```python
from build123d import *

# Parameters (mm, degrees)
CYLINDER003_R     = 2.5
CYLINDER003_DEPTH = 10
CYLINDER_R        = 5
CYLINDER_DEPTH    = 10
CYLINDER002_R     = 2.5
CYLINDER002_DEPTH = 10


with BuildPart() as cylinder003:
    # Cylinder003 → Cylinder003 (new body)
    with BuildSketch(Plane(origin=(-5, 0, 0), x_dir=(0, 0, -1), z_dir=(1, 0, 0))):
        Circle(CYLINDER003_R)
    extrude(amount=CYLINDER003_DEPTH)


with BuildPart() as cut001:
    # Cylinder → Cylinder (new body)
    with BuildSketch(Plane(origin=(-5, 0, 0), x_dir=(0, 0, -1), z_dir=(1, 0, 0))):
        Circle(CYLINDER_R)
    extrude(amount=CYLINDER_DEPTH)

    # Cut001: cut Cylinder003
    add(cylinder003.part, mode=Mode.SUBTRACT)


with BuildPart() as cylinder002:
    # Cylinder002 → Cylinder002 (new body)
    with BuildSketch(Plane(origin=(-5, 0, 0), x_dir=(0, 0, -1), z_dir=(1, 0, 0))):
        Circle(CYLINDER002_R)
    extrude(amount=CYLINDER002_DEPTH)


with BuildPart() as fusion:
    # Sketch → Revolve (revolve)
    with BuildSketch(Plane.XY):
        Polygon((-4.4, 0), (-4.4, 7.615), (-3, 9.015), (3, 9.015), (4.4, 7.615), (4.4, 0), (0, 0), align=None)
    revolve(axis=Axis((0, 0, 0), (1, 0, 0)))

    # Cut: cut Cylinder002
    add(cylinder002.part, mode=Mode.SUBTRACT)

    # Fusion: union Cut001
    add(cut001.part)


solid = fusion.part
```
Geometry: final body of the model. Coordinates: model frame, mm. A direction names the side the tool comes from. Coordinates: 2 decimals unless noted, no trailing zeros. Order: outer loops, then holes, each group sorted by start corner. A loop starts at its lowest first (then second) coordinate and runs counter-clockwise, first axis right, second up. Notation, with made-up numbers: (32.5, 26) - (73.5, 26) arc R18 ccw to (73.5, 61) - close; hole circle Ø11 at (10.25, 21). An arc over 180 degrees is marked (long way). Write each question's results on one line, items separated by ' | '.
1) Section D-D, the plane x = 3.75. Return loops of the section in (y, z) (3 decimals).
Results list:
outline: circle Ø16.53 at (0, 0); hole circle Ø5 at (0, 0)
2) Pull-direction query (Y, two-part tool) for faces 1 (the cylindrical face through (0.04, -7.15, -5.49)), 2 (the cylindrical face through (-0.07, -2.44, 0.54)), 3 (the flat face through (4.4, 2, -5)); classes: pulls with the +Y half, pulls with the -Y half, needs draft (parallel to the pull), parting line crosses it, or undercut.
Results list:
face 1: parting line crosses it | face 2: undercut | face 3: needs draft
3) Section A-A, the plane y = 0. Return loops of the section in (x, z) (3 decimals), plus the area to 3 significant figures.
Results list:
outline: (-5, -5) - (-4.4, -5) - (-4.4, -7.615) - (-3, -9.015) - (3, -9.015) - (4.4, -7.615) - (4.4, -5) - (5, -5) - (5, -2.5) - (-5, -2.5) - close; (-5, 2.5) - (5, 2.5) - (5, 5) - (4.4, 5) - (4.4, 7.615) - (3, 9.015) - (-3, 9.015) - (-4.4, 7.615) - (-4.4, 5) - (-5, 5) - close | area: 117 mm^2
4) Set-up query: faces 4 (the flat face through (-5, -2, -2)), 5 (the cylindrical face through (4.7, -4.88, 1.08)), 6 (the flat face through (-4.4, -2, -5)). Return all of +Z, -Z, +X, -X, +Y, -Y with unobstructed straight access to the full face (end or side cutting, diameter ignored); none if empty.
Results list:
face 4: +Z, -Z, -X, +Y, -Y | face 5: +X | face 6: -X
5) Section C-C, the plane x = 2. Return loops of the section in (y, z) (3 decimals).
Results list:
outline: circle Ø18.03 at (0, 0); hole circle Ø5 at (0, 0)
6) Line query: line 1 (Y direction, x = -4.5, z = 4); line 2 (X direction, y = 5.5, z = 1.25); line 3 (Y direction, x = -3.5, z = 0.75). Output: solid intervals per line, ascending. Write a range as from..to.
Results list:
line 1: -3..3 | line 2: -4.4..4.4 | line 3: -8.48..-2.38, 2.38..8.48
7) Pin query (flat end, axial travel): pin 1 (4 mm diameter, centred on x = 3.5, z = 3, fed in from +Y); pin 2 (2 mm diameter, centred on x = 2.5, z = 5, fed in from -Y); pin 3 (1 mm diameter, centred on x = 2.5, y = -3.5, fed in from +Z). Return the tip coordinate at first contact, or that it passes through.
Results list:
pin 1: y = 8.95 | pin 2: y = -8.08 | pin 3: z = 8.5
